Autodesk Inventor part; units mm, degrees
ref_plane "YZ Plane" through (0, 0, 0) normal (1, 0, 0) x (0, 1, 0)
ref_plane "XZ Plane" through (0, 0, 0) normal (0, 1, 0) x (-1, 0, 0)
ref_plane "XY Plane" through (0, 0, 0) normal (0, 0, 1) x (1, 0, 0)
sketch "Skizze1" plane through (0, 0, 0) normal (0, 0, 1) x (1, 0, 0)
  circle A0 centre (0, 0) radius 6.5
  circle A1 centre (0, 0) radius 9.5
  dimension "d0" = 13
  dimension "d1" = 19
extrude "Extrusion1" add sketch "Skizze1" along normal blind 1.25
sketch "Skizze2" plane through (0, 0, 1.25) normal (0, 0, 1) x (1, 0, 0)
  circle A0 centre (0, 0) radius 6.5
  circle A1 centre (0, 0) radius 7.5
  dimension "d4" = 15
extrude "Extrusion2" add sketch "Skizze2" along normal blind 6.4
sketch "Skizze3" plane through (0, 0, 7.65) normal (0, 0, 1) x (1, 0, 0)
  circle A0 centre (0, 0) radius 6.5
  circle A1 centre (0, 0) radius 9.5
extrude "Extrusion3" add sketch "Skizze3" along normal blind 1.25
fillet "Rundung1" radius 2 2 edges at (-9.5, 0, 7.65) (-9.5, 0, 1.25)
properties part number "Prusa_pulley"
Geometry: final body of the model. Coordinates: model frame, mm. Give positions to 0.01 mm unless a question says otherwise; leave off trailing zeros. Loops run counter-clockwise (first coordinate to the right, second up) from the corner with the lowest first, then second, coordinate; pieces in that order, holes last. Notation, with made-up numbers: (61.25, -15.75) -> (70.25, -15.75) arc R27 ccw to (70.25, 3.25) -> close; hole circle Ø8 at (-35.5, 11.25). An arc over 180 degrees is marked (long way). Put each result on its own line as item: value.
1. Cut plane A-A (y = 0). Return the cut outline in (x, z).
Taken from the geometry:
outline: (-9.5, 0) -> (-6.5, 0) -> (-6.5, 8.9) -> (-9.5, 8.9) arc R2 ccw to (-7.65, 7.65) -> (-7.5, 7.65) -> (-7.5, 1.25) -> (-7.65, 1.25) arc R2 ccw to start; (6.5, 0) -> (9.5, 0) arc R2 ccw to (7.65, 1.25) -> (7.5, 1.25) -> (7.5, 7.65) -> (7.65, 7.65) arc R2 ccw to (9.5, 8.9) -> (6.5, 8.9) -> close
2. Cut plane C-C (z = 4.5). Return the cut outline in (x, y), plus the area to 3 significant figures.
Taken from the geometry:
outline: circle Ø15 at (0, 0); hole circle Ø13 at (0, 0)
area: 44.0 mm2
3. Pin query (flat end, axial travel): P1, Ø1, axis at y = -5.5, z = 6, coming from the -X side; P2, Ø1, axis at y = -2.5, z = 7.5, coming from the -X side; P3, Ø1, axis at y = 3.5, z = 7, coming from the +X side; P4, Ø1, axis at x = -7, y = 0.5, coming from the -Z side. Return the tip coordinate at first contact, or that it passes through.
Taken from the geometry:
P1: stops at x = -5.59
P2: stops at x = -8.43
P3: stops at x = 6.87
P4: stops at z = 0
4. Pull-direction query (X, two-part tool) for faces 1 (the cylindrical face through (-7.493, -0.33, 4.405)), 2 (the flat face through (4, -6, 8.9)), 3 (the cylindrical face through (-5.158, 3.955, 4.388)); classes: released by +X, released by -X, zero draft, split by the parting line, or undercut.
Taken from the geometry:
face 1: split by the parting line
face 2: zero draft
face 3: undercut
5. Ray query, line 1 along Y through (x, z) = (0, 4); line 2 along Z through (x, y) = (7.75, 0.25); line 3 along Y through (x, z) = (2.25, 2.5). Return the intervals inside material, ascending. Write a range as [from, to].
Taken from the geometry:
line 1: y = [-7.5, -6.5], [6.5, 7.5]
line 2: z = [0, 1.25], [7.65, 8.9]
line 3: y = [-7.15, -6.1], [6.1, 7.15]
